Autodesk Inventor part; units mm, degrees
ref_plane "Plano de trabalho1" through (0, 0, 30) normal (0, 0, 1) x (1, 0, 0)
ref_plane "Plano de trabalho2" through (40, 0, 0) normal (1, 0, 0) x (0, 1, 0)
ref_plane "XZ Plane" through (0, 0, 0) normal (0, 1, 0) x (-1, 0, 0)
sketch "Esboço1" plane through (0, 0, 0) normal (0, 0, 1) x (1, 0, 0)
  circle A0 centre (0, 0) radius 30
  circle A1 centre (0, 0) radius 40
  dimension "d0" = 60
  dimension "d1" = 80
extrude "Extrusão1" add sketch "Esboço1" along normal blind 60
sketch "Esboço2" plane through (0, 0, 60) normal (0, 0, 1) x (1, 0, 0)
  circle A0 centre (-50, 0) radius 4
  arc A1 (-50, 8) -> (-50, -8) centre (-50, 0) ccw
  line L0 (-50, 8) -> (-39.1918, 8)
  circle A2 centre (0, 0) radius 40
  line L1 (-50, -8) -> (-39.1918, -8)
  arc A3 (-39.1918, 8) -> (-39.1918, -8) centre (0, 0) ccw
  dimension "d4" = 8
  dimension "d5" = 16
  dimension "d6" = 50
extrude "Extrusão2" add sketch "Esboço2" against normal blind 10 contours L0 A2 L1 A1
pattern_circular "Padrão circular1" count 3 over 360 about axis through (0, 0, 0) along (0, 0, 1) of "Extrusão2"
ref_plane "Plano de trabalho1" through (0, 0, 30) normal (0, 0, 1) x (1, 0, 0)
mirror "Espelhamento1" about plane through (0, 0, 30) normal (0, 0, 1) of "Extrusão2", "Padrão circular1", "Extrusão1"
ref_plane "Plano de trabalho2" through (40, 0, 0) normal (1, 0, 0) x (0, 1, 0)
sketch "Esboço3" plane through (40, 0, 0) normal (1, 0, 0) x (0, 1, 0)
  line L0 (0, 0) -> (0, 60) construction
  line L1 (-4, 60) -> (4, 60) construction
  circle A0 centre (0, 30) radius 25
  dimension "d14" = 50
extrude "Extrusão3" add sketch "Esboço3" along normal blind 5 and the other way blind 10
sketch "Esboço4" plane through (45, 0, 30) normal (1, 0, 0) x (0, 0, -1)
  circle A0 centre (0, 0) radius 8
  point P0 (30, 0)
  dimension "d19" = 16
extrude "Extrusão4" cut sketch "Esboço4" against normal up to next
sketch "Esboço5" plane through (45, 0, 30) normal (1, 0, 0) x (0, 0, -1)
  circle A0 centre (0, 0) radius 14
  circle A1 centre (0, 0) radius 8
  point P0 (30, 0)
  dimension "d22" = 28
  dimension "d23" = 16
extrude "Extrusão5" cut sketch "Esboço5" against normal blind 5
sketch "Esboço6" plane through (45, 0, 30) normal (1, 0, 0) x (0, 0, -1)
  circle A0 centre (0, 0) radius 14 construction
  line L0 (14, 0) -> (25, 0) construction
  circle A1 centre (0, 0) radius 25 construction
  circle A2 centre (19.5, 0) radius 2.25
  point P0 (30, 0)
  dimension "d26" = 4.5
extrude "Extrusão6" cut sketch "Esboço6" against normal blind 10
pattern_circular "Padrão circular2" count 3 over 360 about axis through (45, 0, 30) along (-1, 0, 0) of "Extrusão6"
thread "Rosca1"
thread "Rosca2"
thread "Rosca3"
properties part number "Corpo da Valvula"
CAD build for the part. Positions are in the model's coordinates, mm. A direction names the side the tool comes from. Round coordinates to 2 decimals unless told otherwise and drop trailing zeros. Write each loop counter-clockwise with the first axis right and the second up, starting at its lowest first coordinate (ties: lowest second). Pieces come first, ordered by that corner, then holes. Notation, with made-up numbers: (65, -13) -> (83, -13) arc R20 cw to (83, 6) -> close; hole circle Ø4 at (87.25, 36). An arc over 180 degrees is marked (long way). Answer in a Markdown table with one row per item. Add a question column.
Item 1: Saw through at A-A, the plane x = -24. Write the cut outline in (y, z).
Item 2: Saw through at D-D, the plane x = -48. Write the cut outline in (y, z).
Item 3: Drill centre lines: line 1 (Y direction, x = -50, z = 6); line 2 (Z direction, x = -47, y = -5.5); line 3 (X direction, y = -26, z = 23.5). Where is each one in solid material? Low to high. Write a range as from..to.
Item 4: Drop flat-ended pins along their axis: pin 1 Ø1.5 at (x, z) = (-24, 36) entering from +Y; pin 2 Ø8 at (x, z) = (-4, 48.5) entering from -Y; pin 3 Ø6 at (y, z) = (-16.89, 39.75) entering from -X; pin 4 Ø8 at (x, y) = (-24, -40.5) entering from -Z. Give the stop position or say it passes through.
Item 5: Which spindle directions (+Z, -Z, +X, -X, +Y, -Y) get a long thin tool onto all of the face, cutting with end or side? Do faces 4 (the face through (40.07, 18.785, 38.54)), 5 (the face through (-45, -8, 5)), 6 (the face through (25, 39, 10)), 7 (the face through (29.19, -34.56, 4.93)), 8 (the face through (15.332, 42.556, 4.93)). Say none if no direction does.
Item 6: Mould opens along X. For faces 1 (the face through (-20, 23, 60)), 2 (the face through (24.1, 47.2, 4.9)), 3 (the face through (35, 0, 11)) say: pulls with the +X half, pulls with the -X half, needs draft (parallel to the pull), parting line crosses it, or undercut.
Item 7: Saw through at B-B, the plane y = 12. Write the cut outline in (x, z), then the cut area to 3 significant figures.
Item 8: Saw through at C-C, the plane z = 30. Write the cut outline in (x, y), then the cut area to 3 significant figures.
Findings below:
| question | item | result |
|---|---|---|
| 1 | outline | (-32, 0) -> (-18, 0) -> (-18, 60) -> (-32, 60) -> close; (18, 0) -> (32, 0) -> (32, 60) -> (18, 60) -> close |
| 2 | outline | (-8, 0) -> (-3.46, 0) -> (-3.46, 10) -> (-8, 10) -> close; (-8, 50) -> (-3.46, 50) -> (-3.46, 60) -> (-8, 60) -> close; (3.46, 0) -> (8, 0) -> (8, 10) -> (3.46, 10) -> close; (3.46, 50) -> (8, 50) -> (8, 60) -> (3.46, 60) -> close |
| 3 | line 1 | y = -8..-4, 4..8 |
| 3 | line 2 | z = 0..10, 50..60 |
| 3 | line 3 | x = -30.4..-14.97, 14.97..30.4 |
| 4 | pin 1 | stops at y = 32.55 |
| 4 | pin 2 | stops at y = -40 |
| 4 | pin 3 | stops at x = -37.51 |
| 4 | pin 4 | passes through |
| 5 | face 4 | +X |
| 5 | face 5 | +Z, -Z, -X, -Y |
| 5 | face 6 | +X, +Y |
| 5 | face 7 | +Z, -Z, +X |
| 5 | face 8 | +Z, -Z, +Y |
| 6 | face 1 | needs draft |
| 6 | face 2 | undercut |
| 6 | face 3 | pulls with the +X half |
| 7 | outline | (-38.16, 0) -> (-27.5, 0) -> (-27.5, 60) -> (-38.16, 60) -> close; (27.5, 0) -> (38.16, 0) -> (38.16, 8.07) -> (45, 8.07) -> (45, 22.79) -> (40, 22.79) -> (40, 37.21) -> (45, 37.21) -> (45, 51.93) -> (38.16, 51.93) -> (38.16, 60) -> (27.5, 60) -> close |
| 7 | area | 1,510 mm^2 |
| 8 | outline | (28.91, -8) arc R30 cw (long way) to (28.91, 8) -> (40, 8) -> (40, 14) -> (45, 14) -> (45, 25) -> (31.22, 25) arc R40 ccw (long way) to (31.22, -25) -> (45, -25) -> (45, -14) -> (40, -14) -> (40, -8) -> close |
| 8 | area | 2,280 mm^2 |
